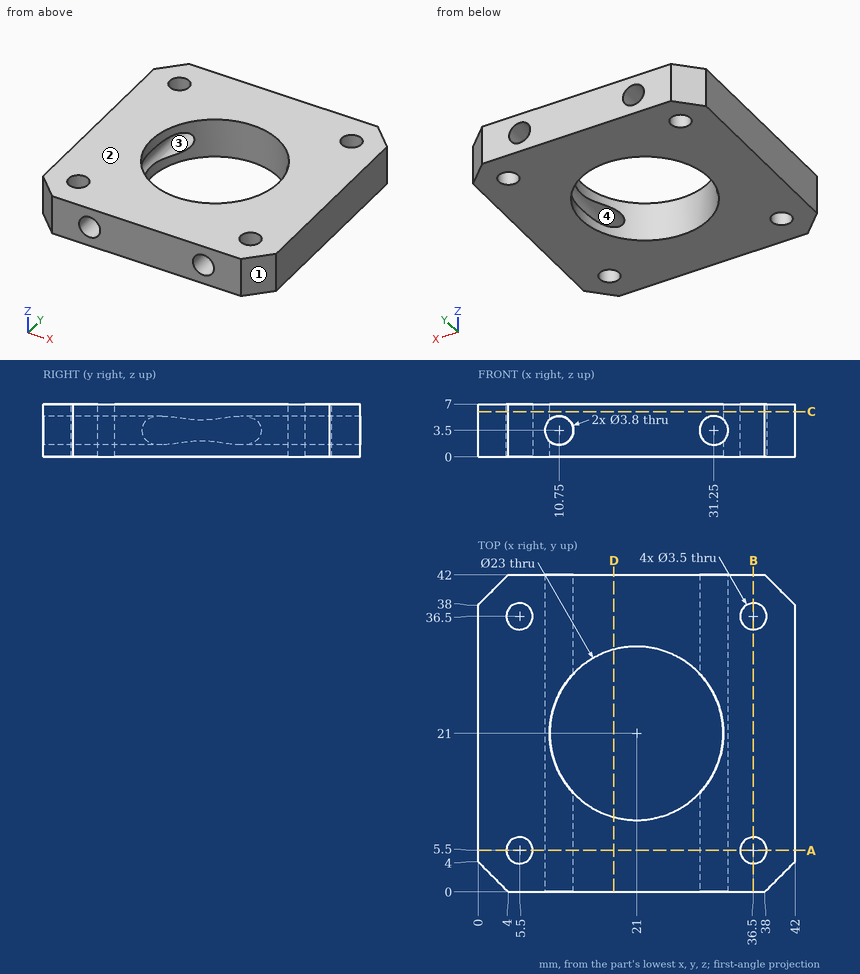
Can you work these out from the drawing? Everything is in mm from the part's minimum corner. Round coordinates to 2 decimals unless told otherwise and drop trailing zeros. Order: outer loops, then holes, each group sorted by start corner. A loop starts at its lowest first (then second) coordinate and runs counter-clockwise, first axis right, second up. Notation, with made-up numbers: (-26, 80.25) -> (-4, 80.25) arc R8 cw to (-4, 93.25) -> close; hole circle Ø7 at (-16, 50). An arc over 180 degrees is marked (long way). Return JSON: item names as keys, results as strings. Group by question number.
1. If we section it at B-B, the plane x = 36.5: Write out the boundary of the cut face in (y, z), then the cut area to 3 significant figures.
2. If we section it at C-C, the plane z = 6: Write out the boundary of the cut face in (x, y), then the cut area to 3 significant figures.
3. If we section it at D-D, the plane x = 18: Write out the boundary of the cut face in (y, z), then the cut area to 3 significant figures.
4. If we section it at A-A, the plane y = 5.5: Write out the boundary of the cut face in (x, z), then the cut area to 3 significant figures.
5. I need wall thicknesses on line 1 (Y direction, x = 36.5, z = 4); line 2 (X direction, y = 33, z = 3.25); line 3 (Y direction, x = 21, z = 5.75). Which ranges of each line are inside material? Lowest first, please. Write a range as [from, to].
6. We'd pull the mould along Z, two halves only. Please class the marked faces 1, 2, 3 and 4: released by +Z, released by -Z, zero draft, split by the parting line, or undercut.
Output values:
{
 "1": {"outline": "(0, 0) -> (3.75, 0) -> (3.75, 7) -> (0, 7) -> close; (7.25, 0) -> (34.75, 0) -> (34.75, 7) -> (7.25, 7) -> close; (38.25, 0) -> (42, 0) -> (42, 7) -> (38.25, 7) -> close", "area": "245 mm²"},
 "2": {"outline": "(0, 4) -> (4, 0) -> (38, 0) -> (42, 4) -> (42, 38) -> (38, 42) -> (4, 42) -> (0, 38) -> close; hole circle Ø3.5 at (5.5, 5.5); hole circle Ø3.5 at (5.5, 36.5); hole circle Ø23 at (21, 21); hole circle Ø3.5 at (36.5, 5.5); hole circle Ø3.5 at (36.5, 36.5)", "area": "1,280 mm²"},
 "3": {"outline": "(0, 0) -> (9.9, 0) -> (9.9, 7) -> (0, 7) -> close; (32.1, 0) -> (42, 0) -> (42, 7) -> (32.1, 7) -> close", "area": "139 mm²"},
 "4": {"outline": "(0, 0) -> (3.75, 0) -> (3.75, 7) -> (0, 7) -> close; (7.25, 0) -> (34.75, 0) -> (34.75, 7) -> (7.25, 7) -> close; (38.25, 0) -> (42, 0) -> (42, 7) -> (38.25, 7) -> close; hole circle Ø3.8 at (10.75, 3.5); hole circle Ø3.8 at (31.25, 3.5)", "area": "222 mm²"},
 "5": {"line 1": "[0, 3.75], [7.25, 34.75], [38.25, 42]", "line 2": "[0, 8.87], [12.63, 29.37], [33.13, 42]", "line 3": "[0, 9.5], [32.5, 42]"},
 "6": {"face 1": "zero draft", "face 2": "released by +Z", "face 3": "undercut", "face 4": "undercut"}
}
